Work out the finished part from the listing and answer in its coordinate system (mm). Face numbers are marked on the shaded views. A direction names the side the tool comes from. Coordinates: 2 decimals unless noted, no trailing zeros. Order: outer loops, then holes, each group sorted by start corner. A loop starts at its lowest first (then second) coordinate and runs counter-clockwise, first axis right, second up. Notation, with made-up numbers: M 76,81 L 84,81 A11 ccw 84,90 Z; hole C 35.25,-33 d10. An arc over 180 degrees is marked long. Answer in a Markdown table with one row per item. Add a question column.
Item 1: Which of the six approach directions +Z, -Z, +X, -X, +Y, -Y give full straight-line access (tool end or side, diameter ignored) to the marked faces 1, 2, 3 and 4?
Item 2: The part is cut by section D-D (x = 32). Write down the section's boundary in (y, z).
Item 3: The part is cut by section C-C (y = -6.75). Write down the section's boundary in (x, z), then the cut area to 3 significant figures.
Item 4: Flat-ended cylindrical pins translate along their axes: pin 1 Ø5 at (x, y) = (11, -1) entering from +Z; pin 2 Ø12 at (x, z) = (21.5, 19) entering from -Y; pin 3 Ø1.8 at (x, y) = (20, 0) entering from +Z. Find the tip coordinate at first contact, or state that the pin passes through.
Item 5: The part is cut by section B-B (z = 26.5). Write down the section's boundary in (x, y), then the cut area to 3 significant figures.
Item 6: Consider line 1 (Z direction, x = 12, y = 0.75); line 2 (X direction, y = 7.25, z = 19); line 3 (Z direction, x = 12, y = 8) (3 decimals). Determine where each line is inside the solid, lowest interval first. Write a range as from..to.
Item 7: The part is cut by section A-A (x = 48). Write down the section's boundary in (y, z).
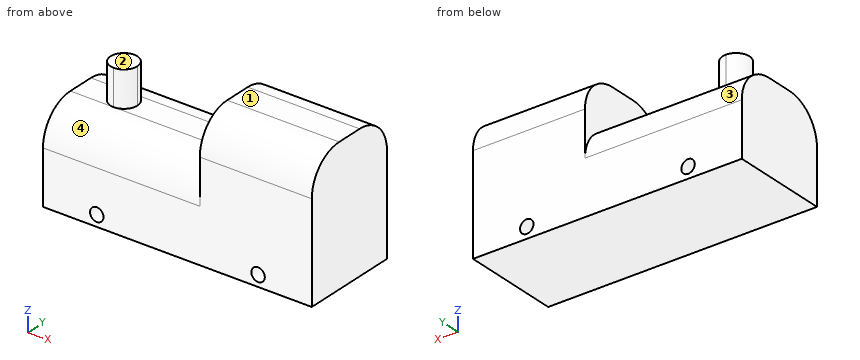
from build123d import *

# Parameters (mm, degrees)
F0_W     = 35
F0_H     = 20
F0_W_2   = 25
F0_H_2   = 10
F1_DEPTH = 11
F2_R     = 8
F3_R     = 8
F5_DEPTH = 8
F6_R     = 1.5
F7_DEPTH = 12.5


# Not quite as in the source:
# - a pattern or mirror of a feature is missing from the dataset's text; its kind, count and spacing are read off the source's solid


with BuildPart() as f1:
    # F0 (on Front) → F1 (new body, symmetric)
    with BuildSketch(Plane.XZ):
        with Locations((17.5, 10)):
            Rectangle(F0_W, F0_H)
        with Locations((47.5, 10)):
            Rectangle(F0_W_2, F0_H)
        with Locations((47.5, 25)):
            Rectangle(F0_W_2, F0_H_2)
    extrude(amount=F1_DEPTH, both=True)

    # F2
    f2_edges = [f1.edges().sort_by_distance(p)[0] for p in [
        (17.5, -11, 20),
        (17.5, 11, 20),
    ]]
    fillet(f2_edges, radius=F2_R)

    # F3
    f3_edges = [f1.edges().sort_by_distance(p)[0] for p in [
        (47.5, -11, 30),
        (47.5, 11, 30),
    ]]
    fillet(f3_edges, radius=F3_R)

    # F4 (on face) → F5 (join)
    with BuildSketch(Plane.XY.offset(20)):
        with BuildLine():
            ThreePointArc((9.6768597141, -3), (11.7981800577, -2.1213203436), (12.6768597141, 0))
            ThreePointArc((12.6768597141, 0), (11.7981800577, 2.1213203436), (9.6768597141, 3))
            ThreePointArc((9.6768597141, 3), (6.6768597141, 0), (9.6768597141, -3))
        make_face()
    extrude(amount=F5_DEPTH)

    # F6 (on Front) → F7 (cut, symmetric)
    with BuildSketch(Plane.XZ):
        with Locations((12, 2.5)):
            Circle(F6_R)
    f7 = extrude(amount=F7_DEPTH, both=True, mode=Mode.SUBTRACT)

    # F7_copies: F7 across plane
    add(f7.mirror(Plane(origin=(30, 0, 0), x_dir=(0, 0, 1), z_dir=(1, 0, 0))), mode=Mode.SUBTRACT)


solid = f1.part
Reply:
| question | item | result |
|---|---|---|
| 1 | face 1 | +Z, +X, -X, +Y, -Y |
| 1 | face 2 | +Z, -X, +Y, -Y |
| 1 | face 3 | +Z, -X, +Y |
| 1 | face 4 | +Z, -X, -Y |
| 2 | outline | M -11,0 L 11,0 L 11,12 A8 ccw 3,20 L -3,20 A8 ccw -11,12 Z |
| 3 | outline | M 0,0 L 60,0 L 60,29.07 L 35,29.07 L 35,19.07 L 0,19.07 Z; hole C 12,2.5 d3; hole C 48,2.5 d3 |
| 3 | area | 1,380 mm2 |
| 4 | pin 1 | stops at z = 28 |
| 4 | pin 2 | stops at y = -10.94 |
| 4 | pin 3 | stops at z = 20 |
| 5 | outline | C 9.68,0 d6; M 35,-9.61 L 60,-9.61 L 60,9.61 L 35,9.61 Z |
| 5 | area | 509 mm2 |
| 6 | line 1 | z = 0..1, 4..28 |
| 6 | line 2 | x = 35..60 |
| 6 | line 3 | z = 0..1, 4..18.245 |
| 7 | outline | M -11,0 L 11,0 L 11,1 L -11,1 Z; M -11,4 L 11,4 L 11,22 A8 ccw 3,30 L -3,30 A8 ccw -11,22 Z |
